from build123d import *

# Parameters (mm, degrees)
BOSS_EXTRUDE1_DEPTH                = 914.4
BOSS_EXTRUDE1_DEPTH_BACK           = 914.4
SKETCH3_W                          = 25.4
SKETCH3_H                          = 25.4
SKETCH3_W_2                        = 22.225
SKETCH3_H_2                        = 22.225
SKETCH5_W                          = 30.406422512
SKETCH5_H                          = 27.345599006
CUT_EXTRUDE1_DEPTH                 = 1117.6
F_1_4_0_25_DIAMETER_HOLE1_D        = 6.35
F_3_16_0_1875_DIAMETER_HOLE1_D     = 4.7625
F_3_16_0_1875_DIAMETER_HOLE1_DEPTH = 1.5875
F_10_CLEARANCE_HOLE1_D             = 5.1054
F_10_CLEARANCE_HOLE1_DEPTH         = 1.5875


with BuildPart() as part:
    # Sketch3 → Boss-Extrude1 (new, two sides: drawn at the far end of the back side and taken through both)
    with BuildSketch(Plane.XY.offset(-BOSS_EXTRUDE1_DEPTH_BACK)):
        Rectangle(SKETCH3_W, SKETCH3_H)
        Rectangle(SKETCH3_W_2, SKETCH3_H_2, mode=Mode.SUBTRACT)
    extrude(amount=BOSS_EXTRUDE1_DEPTH + BOSS_EXTRUDE1_DEPTH_BACK)

    # Sketch5 → Cut-Extrude1 (cut)
    with BuildSketch(Plane.XY.offset(914.4)):
        Rectangle(SKETCH5_W, SKETCH5_H)
    extrude(amount=-CUT_EXTRUDE1_DEPTH, mode=Mode.SUBTRACT)

    # 1/4 (0.25) Diameter Hole1 (through all)
    with Locations(Plane.ZY.offset(12.7)):
        with Locations((-736.6, 0)):
            Hole(F_1_4_0_25_DIAMETER_HOLE1_D / 2)

    # 3/16 (0.1875) Diameter Hole1
    with Locations(Plane(origin=(0, -12.7, 0), x_dir=(-1, 0, 0), z_dir=(0, -1, 0))):
        with Locations((0, 889), (0, 863.6), (0, 838.2), (0, 279.4), (0, 254), (0, 228.6)):
            Hole(F_3_16_0_1875_DIAMETER_HOLE1_D / 2, depth=F_3_16_0_1875_DIAMETER_HOLE1_DEPTH)

    # #10 Clearance Hole1
    with Locations(Plane(origin=(0, -12.7, 0), x_dir=(-1, 0, 0), z_dir=(0, -1, 0))):
        with Locations((0, 635), (0, 584.2), (0, 533.4), (0, 482.6)):
            Hole(F_10_CLEARANCE_HOLE1_D / 2, depth=F_10_CLEARANCE_HOLE1_DEPTH)


solid = part.part
The model under review builds one solid part; all positions refer to its coordinate system, in mm. A direction names the side the tool comes from. Round coordinates to 2 decimals unless told otherwise and drop trailing zeros. Loops run counter-clockwise (first coordinate to the right, second up) from the corner with the lowest first, then second, coordinate; pieces in that order, holes last. Notation, with made-up numbers: (30, 82.5) -> (54, 82.5) arc R17 cw to (54, 105.5) -> close; hole circle Ø3 at (58.5, 82). An arc over 180 degrees is marked (long way). Write item = value, one per line. Start each with the question number.
Item 1: For faces 4 (the flat face through (-11.3, 0.1, -914.4)), 5 (the flat face through (0, -11.112, -564)), list the 3-axis set-ups (+Z, -Z, +X, -X, +Y, -Y) from which the entire face can be reached by the end or side of a thin tool; tool diameter is ignored.
Item 2: Mouldability with a two-part tool opening along Y and no side actions: class faces 1 (the flat face through (0, -12.7, -564)), 2 (the flat face through (12.7, 0, -564)), 3 (the flat face through (11.112, 0, -564)) as released by +Y, released by -Y, zero draft, split by the parting line, or undercut.
Item 3: Insertion check: pin 1 (3 mm diameter, centred on x = 0, z = -482.6, fed in from -Y); pin 2 (5.5 mm diameter, centred on y = 0, z = -736.6, fed in from -X). Each pin has a flat end and moves straight along its axis. Give the tip position at first contact, or say it passes through.
Item 4: Take a section at A-A on z = -271. Give the boundary of the cut face in (x, y), plus the area to 3 significant figures.
Item 5: To check wall thickness, follow L1, parallel to Y at x = 5.25, z = -264; L2, parallel to X at y = -11.8, z = -228.6. State the ranges of each line that lie inside material, in increasing order.
Result:
q1.face_4 = -Z, +X, -X, +Y, -Y
q1.face_5 = +Z, -Z
q2.face_1 = released by -Y
q2.face_2 = zero draft
q2.face_3 = undercut
q3.pin_1 = 11.11
q3.pin_2 = through
q4.outline = (-12.7, -12.7) -> (12.7, -12.7) -> (12.7, 12.7) -> (-12.7, 12.7) -> close; hole (-11.11, -11.11) -> (11.11, -11.11) -> (11.11, 11.11) -> (-11.11, 11.11) -> close
q4.area = 151 mm²
q5.L1 = -12.7 to -11.11, 11.11 to 12.7
q5.L2 = -12.7 to -2.38, 2.38 to 12.7
